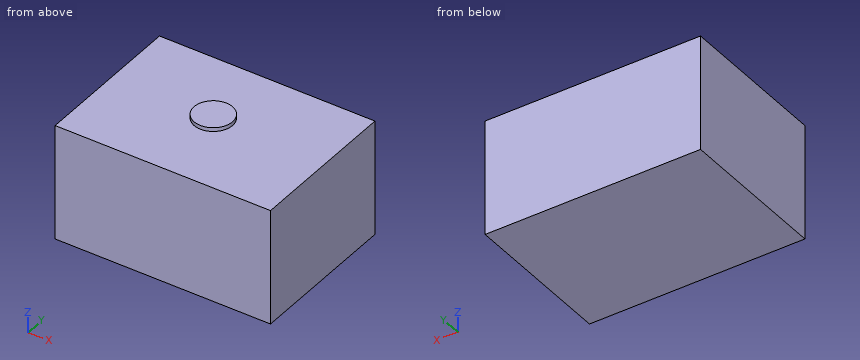
Autodesk Inventor part; units mm, degrees
ref_plane "YZ Plane" through (0, 0, 0) normal (1, 0, 0) x (0, 1, 0)
ref_plane "XZ Plane" through (0, 0, 0) normal (0, 1, 0) x (-1, 0, 0)
ref_plane "XY Plane" through (0, 0, 0) normal (0, 0, 1) x (1, 0, 0)
sketch "Sketch2" plane through (0, 0, 0) normal (0, 0, 1) x (1, 0, 0)
  point P0 (0, 0)
sketch "Sketch3" plane through (0, 0, 0) normal (0, 0, 1) x (1, 0, 0)
  line L0 (0, 0) -> (280, 0)
  line L1 (280, 0) -> (280, 200)
  line L2 (280, 200) -> (0, 200)
  line L3 (0, 200) -> (0, 0)
  dimension "d0" = 280
  dimension "d1" = 200
extrude "Extrusion1" add sketch "Sketch3" along normal blind 150
sketch "Sketch4" plane through (0, 0, 150) normal (0, 0, 1) x (1, 0, 0)
  circle A0 centre (132.9986, 107.0989) radius 25
  point P0 (0, 0)
  dimension "d4" = 50
extrude "Extrusion2" add sketch "Sketch4" along normal blind 5
properties part number "Sensor"
Here's how the part is built. I have some questions about the finished solid (model axes, mm). Coordinates: 2 decimals unless noted, no trailing zeros. Write each loop counter-clockwise with the first axis right and the second up, starting at its lowest first coordinate (ties: lowest second). Pieces come first, ordered by that corner, then holes. Notation, with made-up numbers: (-19, 66) - (40, 66) arc R21 ccw to (40, 105) - close; hole circle Ø3 at (-24, -4). An arc over 180 degrees is marked (long way). One line per item, written item: value.
1) Suppose I cut it at D-D on y = 66. Write out the boundary of the cut face in (x, z), and give its area (3 significant figures).
Model answer:
outline: (0, 0) - (280, 0) - (280, 150) - (0, 150) - close
area: 42,000 mm²
2) I need wall thicknesses on line 1 along Z through (x, y) = (241.5, 70.5). Which ranges of the line are inside material? Lowest first, please.
Model answer:
line 1: z = 0 to 150
3) Suppose I cut it at A-A on x = 161.5. Write out the boundary of the cut face in (y, z).
Model answer:
outline: (0, 0) - (200, 0) - (200, 150) - (0, 150) - close
4) I'm going to push flat-ended pins straight in: P1, Ø3, axis at y = 127, z = 101.5, coming from the -X side; P2, Ø8, axis at x = 165, y = 21, coming from the +Z side. Where does each tip first touch, or does it pass through?
Model answer:
P1: stops at x = 0
P2: stops at z = 150
5) Suppose I cut it at B-B on y = 113.5. Write out the boundary of the cut face in (x, z).
Model answer:
outline: (0, 0) - (280, 0) - (280, 150) - (157.17, 150) - (157.17, 155) - (108.83, 155) - (108.83, 150) - (0, 150) - close
6) Suppose I cut it at C-C on x = 118. Write out the boundary of the cut face in (y, z).
Model answer:
outline: (0, 0) - (200, 0) - (200, 150) - (127.1, 150) - (127.1, 155) - (87.1, 155) - (87.1, 150) - (0, 150) - close
